For this review, take the finished solid that the model builds, in its own axes (mm). A direction names the side the tool comes from. Give positions to 0.01 mm unless a question says otherwise; leave off trailing zeros. Order: outer loops, then holes, each group sorted by start corner. A loop starts at its lowest first (then second) coordinate and runs counter-clockwise, first axis right, second up.
Item 1: Machinability: for faces 1 (the flat face through (-39, -4, -76.35)), 2 (the flat face through (6.3, -3, -4)), 3 (the flat face through (-42, -3, -65)), 4 (the cylindrical face through (-0.177, -4.479, -1.905)), which of the approach directions +Z, -Z, +X, -X, +Y, -Y give a long, thin tool a straight path to every point of the face, cutting with its end or side? Answer none if there is none.
Item 2: Consider section B-B (x = -58). Give the boundary of the cut face in (y, z), plus the area to 3 significant figures.
Item 3: Consider section A-A (z = -67). Give the boundary of the cut face in (x, y), plus the area to 3 significant figures.
Item 4: Consider section C-C (z = 79). Give the boundary of the cut face in (x, y), plus the area to 3 significant figures.
Item 5: The part is to be moulded in two halves that separate along Z. For faces 5 (the cylindrical face through (-23.263, 1.479, 0.637)), 6 (the flat face through (-39, -4, -52.935)), 7 (the cylindrical face through (-124.88, 1.48, -5.5)), say which applies: released by +Z, released by -Z, zero draft, split by the parting line, or undercut.
Item 6: For probe 1 along Z at (x, y) = (-39, -3.75); probe 2 along Y at (x, z) = (84, -70); probe 3 along Z at (x, y) = (21.5, 0.5), list the stretches that pass through material, from the lowest coordinate up.
Item 7: For P1, Ø2.5, axis at y = -5.5, z = -68.5, coming from the +X side; P2, Ø0.9, axis at y = 1.5, z = -94, coming from the +X side; P3, Ø5.5, axis at y = -3.5, z = -66, coming from the -X side, all flat-tipped, find the tip position at first contact; note any pin that passes through.
```python
from build123d import *

# Parameters (mm, degrees)
IZIM1_R                     = 125
IZIM1_W                     = 70
IZIM1_H                     = 72.635569235
Y_KSEKLIK_EKSTR_ZYON1_DEPTH = 3
IZIM6_W                     = 4
IZIM6_H                     = 23.415137081
Y_KSEKLIK_EKSTR_ZYON3_DEPTH = 4
Y_KSEKLIK_EKSTR_ZYON4_START = 4
IZIM6_3_W                   = 7
IZIM6_3_H                   = 23.415137081
Y_KSEKLIK_EKSTR_ZYON4_DEPTH = 3
IZIM8_R                     = 2.5
Y_KSEKLIK_EKSTR_ZYON5_DEPTH = 3
Y_KSEKLIK_EKSTR_ZYON6_START = 3
IZIM8_4_R                   = 4.5
Y_KSEKLIK_EKSTR_ZYON6_DEPTH = 3
KES_EKSTR_ZYON1_DEPTH       = 4


with BuildPart() as part:
    # Çizim1 → Yükseklik-Ekstrüzyon1 (new body)
    with BuildSketch(Plane(origin=(0, 0, 0), x_dir=(1, 0, 0), z_dir=(0, 1, 0))):
        Circle(IZIM1_R)
        with Locations((0, 76.317784617)):
            Rectangle(IZIM1_W, IZIM1_H, mode=Mode.SUBTRACT)
    extrude(amount=Y_KSEKLIK_EKSTR_ZYON1_DEPTH)

    # Çizim6 → Yükseklik-Ekstrüzyon3 (add)
    with BuildSketch(Plane.XZ):
        with Locations((-40, -64.642786203)):
            Rectangle(IZIM6_W, IZIM6_H)
    extrude(amount=Y_KSEKLIK_EKSTR_ZYON3_DEPTH)

    # Çizim6<3> → Yükseklik-Ekstrüzyon4 (add)
    with BuildSketch(Plane.XZ.offset(Y_KSEKLIK_EKSTR_ZYON4_START)):
        with Locations((-38.5, -64.642786203)):
            Rectangle(IZIM6_3_W, IZIM6_3_H)
    extrude(amount=Y_KSEKLIK_EKSTR_ZYON4_DEPTH)

    # Çizim8 → Yükseklik-Ekstrüzyon5 (add)
    with BuildSketch(Plane.XZ):
        with Locations((4.318604625, -2.102613205)):
            Circle(IZIM8_R)
    extrude(amount=Y_KSEKLIK_EKSTR_ZYON5_DEPTH)

    # Çizim8<4> → Yükseklik-Ekstrüzyon6 (add)
    with BuildSketch(Plane.XZ.offset(Y_KSEKLIK_EKSTR_ZYON6_START)):
        with Locations((4.318604625, -2.102613205)):
            Circle(IZIM8_4_R)
    extrude(amount=Y_KSEKLIK_EKSTR_ZYON6_DEPTH)

    # Çizim10 → Kes-Ekstrüzyon1 (cut, through all)
    with BuildSketch(Plane.XZ):
        with BuildLine():
            ThreePointArc((-11.097827728, 1.63805679), (-23.268577728, 0.38383614), (-11.097827728, -0.870384509))
            ThreePointArc((-11.097827728, -0.870384509), (-9.593577728, 0.38383614), (-11.097827728, 1.63805679))
        make_face()
    extrude(amount=-KES_EKSTR_ZYON1_DEPTH, mode=Mode.SUBTRACT)


solid = part.part
```
Resolved:
1. face 1: -Z, +X, -X, -Y
1. face 2: none
1. face 3: +Z, -Z, -X, -Y
1. face 4: -Y
2. outline: (0, -110.73) - (3, -110.73) - (3, 110.73) - (0, 110.73) - close
2. area: 664 mm2
3. outline: (-105.53, 0) - (-42, 0) - (-42, -7) - (-35, -7) - (-35, -4) - (-38, -4) - (-38, 0) - (-35, 0) - (-35, 3) - (-105.53, 3) - close; (35, 0) - (105.53, 0) - (105.53, 3) - (35, 3) - close
3. area: 460 mm2
4. outline: (-96.87, 0) - (96.87, 0) - (96.87, 3) - (-96.87, 3) - close
4. area: 581 mm2
5. face 5: undercut
5. face 6: released by +Z
5. face 7: split by the parting line
6. probe 1: z = -76.35 to -52.94
6. probe 2: y = 0 to 3
6. probe 3: z = -123.14 to -112.64, -40 to 123.14
7. P1: stops at x = -35
7. P2: stops at x = 82.91
7. P3: stops at x = -42
